```python
from build123d import *

# Parameters (mm, degrees)
BASE_FLANGE1_DEPTH     = 2
CUT_EXTRUDE1_START     = -2
CUT_EXTRUDE1_OUTLINE_W = 0.3
CUT_EXTRUDE1_OUTLINE_H = 0.067712434
CUT_EXTRUDE1_DEPTH     = 4
SKETCH8_R              = 0.2
BOSS_EXTRUDE1_DEPTH    = 3.15


# Read off the part's stored shape, not the designer's step: Cut-Extrude1
# Sheet-metal steps are written as plain solids
with BuildPart() as part:
    # Sketch1 → Base-Flange1 (new, symmetric)
    with BuildSketch(Plane(origin=(0, 0, 0), x_dir=(0, 0, -1), z_dir=(1, 0, 0))):
        with BuildLine():
            Line((0, 0), (0, 1.852075023))
            ThreePointArc((0, 1.852075023), (0.09819474, 2.114588994), (0.344567924, 2.24821551))
            Line((0.344567924, 2.24821551), (54.469316873, 9.82191048))
            Line((54.469316873, 9.82191048), (54.51089093, 9.524805115))
            Line((54.51089093, 9.524805115), (0.386141981, 1.951110145))
            ThreePointArc((0.386141981, 1.951110145), (0.324548685, 1.917703516), (0.3, 1.852075023))
            Line((0.3, 1.852075023), (0.3, 0))
            Line((0.3, 0), (0, 0))
        make_face()
    extrude(amount=BASE_FLANGE1_DEPTH, both=True)

    # Cut-Extrude1 outline → Cut-Extrude1 (cut)
    with BuildSketch(Plane(origin=(0, 0, 0), x_dir=(0, 0, -1), z_dir=(1, 0, 0)).offset(CUT_EXTRUDE1_START)):
        with Locations((0.15, 0.033856217)):
            Rectangle(CUT_EXTRUDE1_OUTLINE_W, CUT_EXTRUDE1_OUTLINE_H)
    extrude(amount=CUT_EXTRUDE1_DEPTH, mode=Mode.SUBTRACT)

    # Sketch8 → Boss-Extrude1 (add, symmetric)
    with BuildSketch(Plane(origin=(0, 0, 0), x_dir=(0, 0, -1), z_dir=(1, 0, 0))):
        with Locations((0.15, 0.2)):
            Circle(SKETCH8_R)
    extrude(amount=BOSS_EXTRUDE1_DEPTH, both=True)


solid = part.part
```
Can you work these out from the model? Positions are in its coordinate system, mm. Round coordinates to 2 decimals unless told otherwise and drop trailing zeros. Loops run counter-clockwise (first coordinate to the right, second up) from the corner with the lowest first, then second, coordinate; pieces in that order, holes last.
Item 1: Suppose I cut it at B-B, the plane y = 1.25. Write out the boundary of the cut face in (x, z).
Item 2: If we mould it in two halves opening along Y, with no side actions, what happens to faces 1 (the flat face through (0.03, 5.79, -27.83)), 2 (the flat face through (0, 1, -0.3)), 3 (the flat face through (0, 1, 0))? For each: +Y half, -Y half, draft (parallel to the pull), parting line (faces both ways), or undercut.
Item 3: Will these pins go through, and if not, where does the flat tip stop? pin 1 Ø0.8 at (x, y) = (0, 1) entering from -Z; pin 2 Ø3 at (y, z) = (3.5, -14) entering from -X; pin 3 Ø3 at (y, z) = (6, -34) entering from +X.
Item 4: Please list where these lines run through material, in increasing order: L1, parallel to Z at x = 0, y = 0.75; L2, parallel to Y at x = 0.5, z = -18; L3, parallel to Y at x = -0.25, z = -49.5.
Item 5: Suppose I cut it at C-C, the plane x = -2.5. Write out the boundary of the cut face in (y, z), then the cut area to 3 significant figures.
Item 6: Suppose I cut it at A-A, the plane x = 1.25. Write out the boundary of the cut face in (y, z), then the cut area to 3 significant figures.
Item 7: Suppose I cut it at D-D, the plane z = -50. Write out the boundary of the cut face in (x, y).
Reported:
1. outline: (-2, -0.3) - (2, -0.3) - (2, 0) - (-2, 0) - close
2. face 1: -Y half
2. face 2: undercut
2. face 3: draft
3. pin 1: stops at z = -0.3
3. pin 2: stops at x = -2
3. pin 3: stops at x = 2
4. L1: z = -0.3 to 0
4. L2: y = 4.42 to 4.72
4. L3: y = 8.82 to 9.13
5. outline: circle Ø0.4 at (0.2, -0.15)
5. area: 0.126 mm2
6. outline: (0.33, -0.3) - (1.85, -0.3) arc R0.1 cw to (1.95, -0.39) - (9.52, -54.51) - (9.82, -54.47) - (2.25, -0.34) arc R0.4 ccw to (1.85, 0) - (0.33, 0) arc R0.2 ccw (long way) to start
6. area: 17.1 mm2
7. outline: (-2, 8.89) - (2, 8.89) - (2, 9.2) - (-2, 9.2) - close
